Here's how the part is built. I have some questions about the finished solid (model axes, mm). Face numbers are marked on the shaded views. Round coordinates to 2 decimals unless told otherwise and drop trailing zeros. Order: outer loops, then holes, each group sorted by start corner. A loop starts at its lowest first (then second) coordinate and runs counter-clockwise, first axis right, second up. Notation, with made-up numbers: (31, -13) - (56, -13) arc R13 cw to (56, -8) - close; hole circle Ø4 at (64.25, -18.75). An arc over 180 degrees is marked (long way). Answer as a JSON object with one key per item and string values.
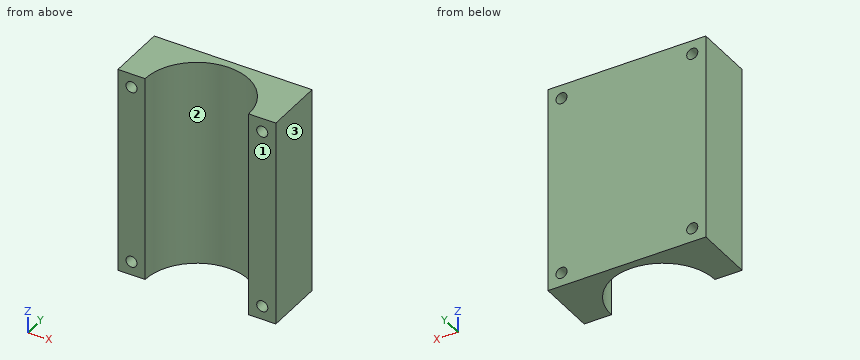
```python
from build123d import *

# Parameters (mm, degrees)
SKETCH1_W                                  = 57.15
SKETCH1_H                                  = 75
BOSS_EXTRUDE1_DEPTH                        = 21.59
CUT_EXTRUDE1_REACH                         = 77
SKETCH5_R                                  = 2.008
CUT_EXTRUDE5_DEPTH                         = 21.59
MIRROR1_AT_THE_SECOND_PLANE_COPY_1_SKETC_R = 2.008
MIRROR1_AT_THE_SECOND_PLANE_COPY_1_DEPTH   = 21.59


with BuildPart() as part:
    # Sketch1 → Boss-Extrude1 (new body)
    with BuildSketch(Plane(origin=(0, 0, 0), x_dir=(1, 0, 0), z_dir=(0, 1, 0))):
        Rectangle(SKETCH1_W, SKETCH1_H)
    extrude(amount=BOSS_EXTRUDE1_DEPTH)

    # Sketch3 → Cut-Extrude1 (cut, up to next)
    with BuildSketch(Plane.XY.offset(37.5), mode=Mode.PRIVATE) as cut_extrude1_sk1:
        with BuildLine():
            Line((-18.75, 0), (18.75, 0))
            ThreePointArc((18.75, 0), (0, 18.75), (-18.75, 0))
        make_face()
    cut_extrude1_tool1 = extrude(cut_extrude1_sk1.sketch, amount=-CUT_EXTRUDE1_REACH, mode=Mode.PRIVATE) & part.part
    add(cut_extrude1_tool1.solids().sort_by_distance((0, 7.957747, 37.5))[0], mode=Mode.SUBTRACT)

    # Sketch5 → Cut-Extrude5 (cut)
    with BuildSketch(Plane(origin=(0, 21.59, 0), x_dir=(1, 0, 0), z_dir=(0, 1, 0))):
        with Locations((-23.6625, -32.5875)):
            Circle(SKETCH5_R)
    cut_extrude5 = extrude(amount=-CUT_EXTRUDE5_DEPTH, mode=Mode.SUBTRACT)

    # Mirror1: Cut-Extrude5 across plane
    add(cut_extrude5.mirror(Plane(origin=(0, 0, 0), x_dir=(0, 0, 1), z_dir=(1, 0, 0))), mode=Mode.SUBTRACT)

    # Mirror1 at the second plane: Cut-Extrude5 across plane
    add(cut_extrude5.mirror(Plane.XY), mode=Mode.SUBTRACT)

    # Mirror1 at the second plane copy 1 sketc → Mirror1 at the second plane copy 1 (cut)
    with BuildSketch(Plane(origin=(0, 21.59, 0), x_dir=(-1, 0, 0), z_dir=(0, 1, 0))):
        with Locations((-23.6625, -32.5875)):
            Circle(MIRROR1_AT_THE_SECOND_PLANE_COPY_1_SKETC_R)
    extrude(amount=-MIRROR1_AT_THE_SECOND_PLANE_COPY_1_DEPTH, mode=Mode.SUBTRACT)


solid = part.part
```
1. If I drill on L1, parallel to X at y = 11, z = 33 (3 decimals); L2, parallel to X at y = 7.25, z = -7 (3 decimals); L3, parallel to Z at x = -23, y = 12.5, over which ranges is the centre line in solid material (lowest first)? Write a range as [from, to].
Responses:
{"L1": "[-28.575, -25.628], [-21.697, -15.184], [15.184, 21.697], [25.628, 28.575]", "L2": "[-28.575, -17.292], [17.292, 28.575]", "L3": "[-37.5, -34.48], [-30.69, 30.69], [34.48, 37.5]"}
2. Imagine slicing it at A-A (y = 6). List the corners of the cut face in (x, z) for me (1 decimal), plus the area to 3 significant figures.
Responses:
{"outline": "(-28.6, -37.5) - (-17.8, -37.5) - (-17.8, 37.5) - (-28.6, 37.5) - close; (17.8, -37.5) - (28.6, -37.5) - (28.6, 37.5) - (17.8, 37.5) - close; hole circle Ø4 at (-23.7, -32.6); hole circle Ø4 at (-23.7, 32.6); hole circle Ø4 at (23.7, -32.6); hole circle Ø4 at (23.7, 32.6)", "area": "1,570 mm2"}
3. Thinking about a two-plate mould opening in X: for the marked faces 1, 2 and 3, which applies, pulls with the +X half, pulls with the -X half, needs draft (parallel to the pull), parting line crosses it, or undercut?
Responses:
{"face 1": "needs draft", "face 2": "undercut", "face 3": "pulls with the +X half"}
4. Imagine slicing it at B-B (z = -9). List the corners of the cut face in (x, y) for me (3 decimals).
Responses:
{"outline": "(-28.575, 0) - (-18.75, 0) arc R18.75 cw to (18.75, 0) - (28.575, 0) - (28.575, 21.59) - (-28.575, 21.59) - close"}
5. For P1, Ø3, axis at x = 23.66, z = 32.59, coming from the -Y side, with a flat end and sliding along its axis, tell me the tip position at first contact or that it passes through.
Responses:
{"P1": "through"}
6. Imagine slicing it at D-D (x = 11.5). List the corners of the cut face in (y, z) for me.
Responses:
{"outline": "(14.81, -37.5) - (21.59, -37.5) - (21.59, 37.5) - (14.81, 37.5) - close"}
7. Imagine slicing it at C-C (y = 11.5). List the corners of the cut face in (x, z) for me (1 decimal), plus the area to 3 significant figures.
Responses:
{"outline": "(-28.6, -37.5) - (-14.8, -37.5) - (-14.8, 37.5) - (-28.6, 37.5) - close; (14.8, -37.5) - (28.6, -37.5) - (28.6, 37.5) - (14.8, 37.5) - close; hole circle Ø4 at (-23.7, -32.6); hole circle Ø4 at (-23.7, 32.6); hole circle Ø4 at (23.7, -32.6); hole circle Ø4 at (23.7, 32.6)", "area": "2,010 mm2"}
